Check sheet for the modelled part. Datum: model origin and axes. Units: mm. A direction names the side the tool comes from. Round coordinates to 2 decimals unless told otherwise and drop trailing zeros. Order: outer loops, then holes, each group sorted by start corner. A loop starts at its lowest first (then second) coordinate and runs counter-clockwise, first axis right, second up. Notation, with made-up numbers: (47, 29.25) -> (100, 29.25) arc R21 ccw to (100, 68.25) -> close; hole circle Ø11 at (-3.5, 13). An arc over 180 degrees is marked (long way). Answer in a Markdown table with one row per item.
from build123d import *

# Parameters (mm, degrees)
CROQUIS1_R              = 6.05
CROQUIS1_R_2            = 1.55
CROQUIS1_R_3            = 9
SALIENTE_EXTRUIR1_DEPTH = 1
CROQUIS1_3_R            = 6.05
CROQUIS1_3_R_2          = 1.55
SALIENTE_EXTRUIR2_DEPTH = 8
CROQUIS2_R              = 9
CROQUIS2_R_2            = 6.05
CROQUIS2_R_3            = 1.55
SALIENTE_EXTRUIR3_DEPTH = 1


with BuildPart() as part:
    # Croquis1 → Saliente-Extruir1 (new body)
    with BuildSketch(Plane(origin=(0, 0, 0), x_dir=(1, 0, 0), z_dir=(0, 1, 0))):
        Circle(CROQUIS1_R)
        Circle(CROQUIS1_R_2, mode=Mode.SUBTRACT)
        Circle(CROQUIS1_R_3)
        Circle(CROQUIS1_R, mode=Mode.SUBTRACT)
    extrude(amount=SALIENTE_EXTRUIR1_DEPTH)

    # Croquis1_3 → Saliente-Extruir2 (add)
    with BuildSketch(Plane(origin=(0, 0, 0), x_dir=(1, 0, 0), z_dir=(0, 1, 0))):
        Circle(CROQUIS1_3_R)
        Circle(CROQUIS1_3_R_2, mode=Mode.SUBTRACT)
    extrude(amount=SALIENTE_EXTRUIR2_DEPTH)

    # Croquis2 → Saliente-Extruir3 (add)
    with BuildSketch(Plane(origin=(0, 8, 0), x_dir=(1, 0, 0), z_dir=(0, 1, 0))):
        Circle(CROQUIS2_R)
        Circle(CROQUIS2_R_2, mode=Mode.SUBTRACT)
        Circle(CROQUIS2_R_2)
        Circle(CROQUIS2_R_3, mode=Mode.SUBTRACT)
    extrude(amount=SALIENTE_EXTRUIR3_DEPTH)


solid = part.part
Item 1: Cross-section at A-A (z = 0). Record the boundary of the cut face in (x, y), and give its area (3 significant figures).
Result sheet:
| item | result |
|---|---|
| outline | (-9, 0) -> (-1.55, 0) -> (-1.55, 9) -> (-9, 9) -> (-9, 8) -> (-6.05, 8) -> (-6.05, 1) -> (-9, 1) -> close; (1.55, 0) -> (9, 0) -> (9, 1) -> (6.05, 1) -> (6.05, 8) -> (9, 8) -> (9, 9) -> (1.55, 9) -> close |
| area | 92.8 mm^2 |
Item 2: Mould release check, pull along X, two halves, no side actions. Record for faces 1 (the flat face through (2, 1, 6)), 2 (the cylindrical face through (0.715, 4.437, 1.375)), 3 (the cylindrical face through (-1.172, 0.493, -8.923)): pulls with the +X half, pulls with the -X half, needs draft (parallel to the pull), parting line crosses it, or undercut.
Result sheet:
| item | result |
|---|---|
| face 1 | needs draft |
| face 2 | undercut |
| face 3 | parting line crosses it |
Item 3: Set-up check for faces 4 (the flat face through (2, 8, 6)), 5 (the cylindrical face through (-1.172, 8.493, -8.923)): record each of +Z, -Z, +X, -X, +Y, -Y from which the full face is reachable in a straight line by a thin tool's end or side.
Result sheet:
| item | result |
|---|---|
| face 4 | none |
| face 5 | +Y, -Y |
Item 4: Cross-section at D-D (z = 5.25). Record the boundary of the cut face in (x, y).
Result sheet:
| item | result |
|---|---|
| outline | (-7.31, 0) -> (7.31, 0) -> (7.31, 1) -> (3.01, 1) -> (3.01, 8) -> (7.31, 8) -> (7.31, 9) -> (-7.31, 9) -> (-7.31, 8) -> (-3.01, 8) -> (-3.01, 1) -> (-7.31, 1) -> close |
Item 5: Cross-section at C-C (y = 8.75). Record the boundary of the cut face in (x, z).
Result sheet:
| item | result |
|---|---|
| outline | circle Ø18 at (0, 0); hole circle Ø3.1 at (0, 0) |
Item 6: Scan lines: line 1 (Z direction, x = 0, y = 3.75); line 2 (Y direction, x = -6.75, z = 5.5). Record each from-to range of solid material in increasing order. Write a range as [from, to].
Result sheet:
| item | result |
|---|---|
| line 1 | z = [-6.05, -1.55], [1.55, 6.05] |
| line 2 | y = [0, 1], [8, 9] |
Item 7: Cross-section at B-B (x = 0). Record the boundary of the cut face in (y, z).
Result sheet:
| item | result |
|---|---|
| outline | (0, -9) -> (1, -9) -> (1, -6.05) -> (8, -6.05) -> (8, -9) -> (9, -9) -> (9, -1.55) -> (0, -1.55) -> close; (0, 1.55) -> (9, 1.55) -> (9, 9) -> (8, 9) -> (8, 6.05) -> (1, 6.05) -> (1, 9) -> (0, 9) -> close |
Item 8: Depth check by flat-ended pin: P1, Ø4, axis at x = -2.5, y = 4, coming from the +Z side; P2, Ø2, axis at y = 1.5, z = 5, coming from the -X side; P3, Ø1.5, axis at x = -4.5, y = 2, coming from the -Z side. Enter the tip coordinate at first touch or a pass-through.
Result sheet:
| item | result |
|---|---|
| P1 | stops at z = 6.03 |
| P2 | stops at x = -7.99 |
| P3 | stops at z = -4.75 |
